The figure shows three views and two pictorial views of one solid part (mm, origin at its lowest corner). Answer the questions. Round coordinates to 2 decimals unless told otherwise and drop trailing zeros. Write each loop counter-clockwise with the first axis right and the second up, starting at its lowest first coordinate (ties: lowest second). Pieces come first, ordered by that corner, then holes. Notation, with made-up numbers: M 82,4.5 L 126,4.5 A16 ccw 126,25.5 Z; hole C -20.5,66.5 d2. An arc over 180 degrees is marked long. One line per item, written item: value. Start each with the question number.
Q1. Find section C-C (z = 13). Write down the section's boundary in (x, y) (1 decimal).
Q2. Find section B-B (y = 17). Write down the section's boundary in (x, z), and give its area (3 significant figures).
Q3. Consider probe 1 along Y at (x, z) = (22.5, 7) (1 decimal); probe 2 along X at (y, z) = (10, 2.25) (1 decimal); probe 3 along X at (y, z) = (21.5, 5.5) (1 decimal). Determine where each line is inside the solid, lowest interval first.
Q4. Given pin 1 Ø12 at (y, z) = (36.5, 20) entering from -X, flat-ended and moving along its own axis, determine where the tip first touches the part or whether it passes through.
Q5. The mould has two halves that part along X. Classify the marked faces 1, 2, 3 and 4: released by +X, released by -X, zero draft, split by the parting line, or undercut.
Q6. Find section A-A (x = 24). Write down the section's boundary in (y, z) (1 decimal).
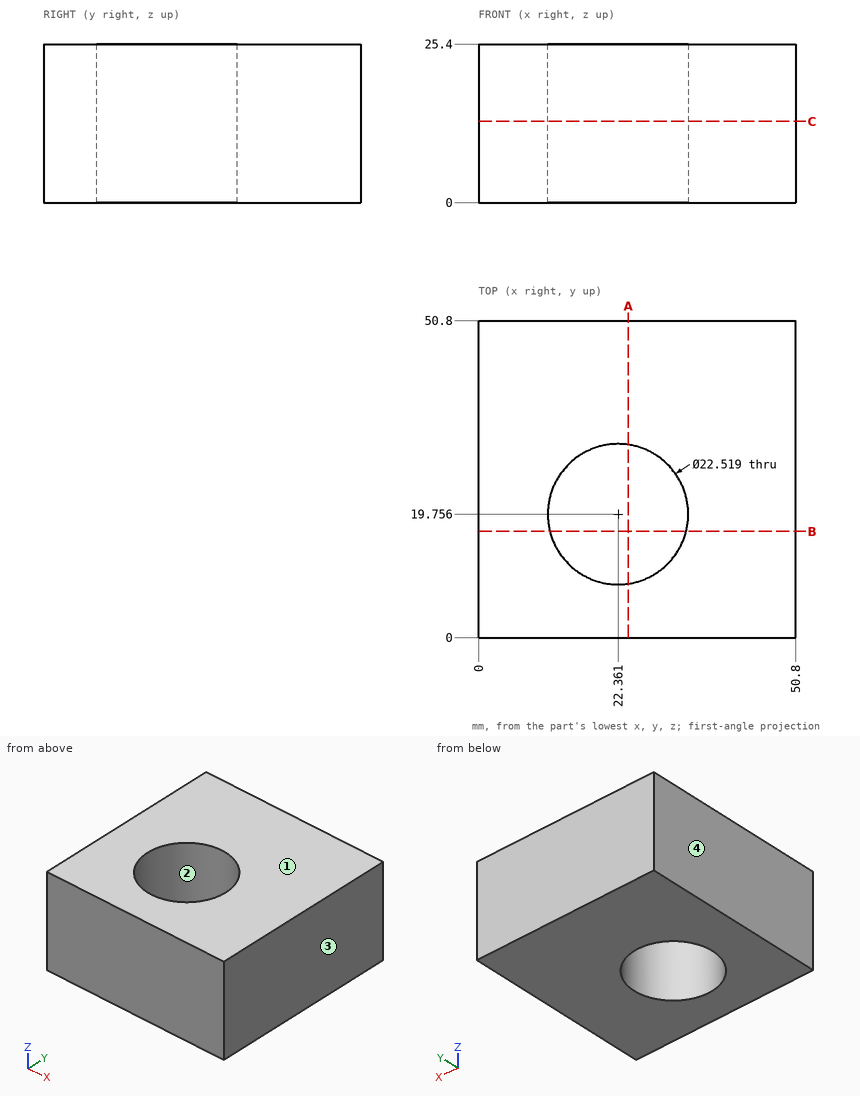
The answers:
1. outline: M 0,0 L 50.8,0 L 50.8,50.8 L 0,50.8 Z; hole C 22.4,19.8 d22.5
2. outline: M 0,0 L 11.44,0 L 11.44,25.4 L 0,25.4 Z; M 33.28,0 L 50.8,0 L 50.8,25.4 L 33.28,25.4 Z
2. area: 736 mm2
3. probe 1: 0 to 8.5, 31 to 50.8
3. probe 2: 0 to 16.7, 28 to 50.8
3. probe 3: 0 to 11.2, 33.5 to 50.8
4. pin 1: x = 0
5. face 1: zero draft
5. face 2: undercut
5. face 3: released by +X
5. face 4: released by -X
6. outline: M 0,0 L 8.6,0 L 8.6,25.4 L 0,25.4 Z; M 30.9,0 L 50.8,0 L 50.8,25.4 L 30.9,25.4 Z
